Here's how the part is built. I have some questions about the finished solid (model axes, mm). A direction names the side the tool comes from. Give positions to 0.01 mm unless a question says otherwise; leave off trailing zeros. Write each loop counter-clockwise with the first axis right and the second up, starting at its lowest first coordinate (ties: lowest second). Pieces come first, ordered by that corner, then holes. Notation, with made-up numbers: (63, -9.5) - (111, -9.5) arc R20 ccw to (111, 29.5) - close; hole circle Ø5 at (29.5, -19.5). An arc over 180 degrees is marked (long way). Use a Markdown table: item, result.
```python
from build123d import *

# Parameters (mm, degrees)
SKETCH1_W           = 50
SKETCH1_H           = 44
BOSS_EXTRUDE1_DEPTH = 5
SKETCH2_W           = 50
SKETCH2_H           = 5
BOSS_EXTRUDE2_DEPTH = 90
SKETCH3_R           = 1.42
CUT_EXTRUDE1_DEPTH  = 60
SKETCH4_R           = 11
CUT_EXTRUDE2_DEPTH  = 2.5
SKETCH5_R           = 3.25
CUT_EXTRUDE3_DEPTH  = 10
SKETCH6_R           = 1.42
CUT_EXTRUDE4_DEPTH  = 10
SKETCH8_W           = 2
SKETCH8_H           = 39
BOSS_EXTRUDE3_DEPTH = 32
CUT_EXTRUDE5_DEPTH  = 35


with BuildPart() as part:
    # Sketch1 → Boss-Extrude1 (new body)
    with BuildSketch(Plane(origin=(0, 0, 0), x_dir=(1, 0, 0), z_dir=(0, 1, 0))):
        Rectangle(SKETCH1_W, SKETCH1_H)
    extrude(amount=BOSS_EXTRUDE1_DEPTH)

    # Sketch2 → Boss-Extrude2 (add)
    with BuildSketch(Plane(origin=(0, 5, 0), x_dir=(1, 0, 0), z_dir=(0, 1, 0))):
        with Locations((0, 19.5)):
            Rectangle(SKETCH2_W, SKETCH2_H)
    extrude(amount=BOSS_EXTRUDE2_DEPTH)

    # Sketch3 → Cut-Extrude1 (cut)
    with BuildSketch(Plane.XY.offset(-17)):
        with Locations((-15.5, 44)):
            Circle(SKETCH3_R)
        with Locations((15.5, 44)):
            Circle(SKETCH3_R)
        with Locations((15.5, 75)):
            Circle(SKETCH3_R)
        with Locations((-15.5, 75)):
            Circle(SKETCH3_R)
    extrude(amount=-CUT_EXTRUDE1_DEPTH, mode=Mode.SUBTRACT)

    # Sketch4 → Cut-Extrude2 (cut)
    with BuildSketch(Plane.XY.offset(-17)):
        with Locations((0, 59.5)):
            Circle(SKETCH4_R)
    extrude(amount=-CUT_EXTRUDE2_DEPTH, mode=Mode.SUBTRACT)

    # Sketch5 → Cut-Extrude3 (cut)
    with BuildSketch(Plane.XY.offset(-19.5)):
        with Locations((0, 59.5)):
            Circle(SKETCH5_R)
    extrude(amount=-CUT_EXTRUDE3_DEPTH, mode=Mode.SUBTRACT)

    # Sketch6 → Cut-Extrude4 (cut)
    with BuildSketch(Plane(origin=(0, 5, 0), x_dir=(1, 0, 0), z_dir=(0, 1, 0))):
        with Locations(Location((-19, 11, 0), (0, 0, 270))):
            Circle(SKETCH6_R)
        with Locations(Location((-19, -16, 0), (0, 0, 270))):
            Circle(SKETCH6_R)
        with Locations(Location((19, -16, 0), (0, 0, 270))):
            Circle(SKETCH6_R)
        with Locations(Location((19, 11, 0), (0, 0, 270))):
            Circle(SKETCH6_R)
    extrude(amount=-CUT_EXTRUDE4_DEPTH, mode=Mode.SUBTRACT)

    # Sketch8 → Boss-Extrude3 (add)
    with BuildSketch(Plane(origin=(0, 5, 0), x_dir=(1, 0, 0), z_dir=(0, 1, 0))):
        with Locations((0, -2.5)):
            Rectangle(SKETCH8_W, SKETCH8_H)
    extrude(amount=BOSS_EXTRUDE3_DEPTH)

    # Sketch9 → Cut-Extrude5 (cut)
    with BuildSketch(Plane(origin=(1, 0, 0), x_dir=(0, 0, -1), z_dir=(1, 0, 0))):
        Polygon((17, 37), (-22, 5), (-22, 37), align=None)
    extrude(amount=-CUT_EXTRUDE5_DEPTH, mode=Mode.SUBTRACT)


solid = part.part
```
Item 1: If we section it at D-D, the plane x = 0: Write out the boundary of the cut face in (y, z), plus the area to 3 significant figures.
Values:
| item | result |
|---|---|
| outline | (0, -22) - (56.25, -22) - (56.25, -19.5) - (48.5, -19.5) - (48.5, -17) - (37, -17) - (5, 22) - (0, 22) - close; (62.75, -22) - (95, -22) - (95, -17) - (70.5, -17) - (70.5, -19.5) - (62.75, -19.5) - close |
| area | 1,220 mm2 |
Item 2: I need wall thicknesses on line 1 along X through (y, z) = (75, -19); line 2 along Y through (x, z) = (-15.5, -20.75); line 3 along X through (y, z) = (4, -11). Which ranges of each line are inside material? Lowest first, please. Write a range as [from, to].
Values:
| item | result |
|---|---|
| line 1 | x = [-25, -16.92], [-14.08, 14.08], [16.92, 25] |
| line 2 | y = [0, 42.58], [45.42, 73.58], [76.42, 95] |
| line 3 | x = [-25, -20.42], [-17.58, 17.58], [20.42, 25] |
Item 3: If we section it at C-C, the plane z = 16: Write out the boundary of the cut face in (x, y), plus the area to 3 significant figures.
Values:
| item | result |
|---|---|
| outline | (-25, 0) - (-20.42, 0) - (-20.42, 5) - (-25, 5) - close; (-17.58, 0) - (17.58, 0) - (17.58, 5) - (1, 5) - (1, 9.92) - (-1, 9.92) - (-1, 5) - (-17.58, 5) - close; (20.42, 0) - (25, 0) - (25, 5) - (20.42, 5) - close |
| area | 231 mm2 |
Item 4: If we section it at B-B, the plane y = 59.5: Write out the boundary of the cut face in (x, z).
Values:
| item | result |
|---|---|
| outline | (-25, -22) - (-3.25, -22) - (-3.25, -19.5) - (-11, -19.5) - (-11, -17) - (-25, -17) - close; (3.25, -22) - (25, -22) - (25, -17) - (11, -17) - (11, -19.5) - (3.25, -19.5) - close |
Item 5: For faces 1 (the flat face through (2.3, 62.1, -19.5)), 2 (the flat face through (-13, 5, 2)), 3 (the flat face through (13, 5, 2)), 4 (the flat face through (-6, 49, -17)), which set-ups out of +Z, -Z, +X, -X, +Y, -Y let a thin tool reach every point of the face, with its end or its side?
Values:
| item | result |
|---|---|
| face 1 | +Z |
| face 2 | +Z, -X, +Y |
| face 3 | +Z, +X, +Y |
| face 4 | +Z, +Y |
Item 6: Will these pins go through, and if not, where does the flat tip stop? pin 1 Ø1 at (x, z) = (-9.5, 10.5) entering from +Y; pin 2 Ø6 at (x, y) = (0.5, 63.5) entering from +Z; pin 3 Ø15 at (x, y) = (7, 72) entering from +Z.
Values:
| item | result |
|---|---|
| pin 1 | stops at y = 5 |
| pin 2 | stops at z = -19.5 |
| pin 3 | stops at z = -17 |
Item 7: Thinking about a two-plate mould opening in X: for faces 5 (the flat face through (-25, 37, -18)), 6 (the cylindrical face through (-15.68, 76.41, -19.46)), 7 (the flat face through (0, 0, 0)), which applies, +X half, -X half, draft (parallel to the pull), parting line (faces both ways), or undercut?
Values:
| item | result |
|---|---|
| face 5 | -X half |
| face 6 | undercut |
| face 7 | draft |
Item 8: If we section it at A-A, the plane x = 15.5: Write out the boundary of the cut face in (y, z), plus the area to 3 significant figures.
Values:
| item | result |
|---|---|
| outline | (0, -22) - (42.58, -22) - (42.58, -17) - (5, -17) - (5, 22) - (0, 22) - close; (45.42, -22) - (73.58, -22) - (73.58, -17) - (45.42, -17) - close; (76.42, -22) - (95, -22) - (95, -17) - (76.42, -17) - close |
| area | 642 mm2 |
